from build123d import *

# Parameters (mm, degrees)
BOSS_EXTRUDE1_DEPTH = 20
CUT_EXTRUDE1_DEPTH  = 59.888175724
CUT_EXTRUDE2_DEPTH  = 79.101263393
HOLE1_D             = 3.4
HOLE2_D             = 3.4
HOLE3_D             = 8.4
HOLE4_D             = 8.4
HOLE5_D             = 8.4
CHAMFER1_SIZE       = 8.485281374
CHAMFER2_SIZE       = 5
CHAMFER3_SIZE       = 8.485281374


with BuildPart() as part:
    # Sketch1 → Boss-Extrude1 (new body)
    with BuildSketch(Plane.XY.offset(20)):
        Polygon((15, -34), (15, -11.339745962), (-2.320508076, 18.660254038), (-21.944863729, 29.990381057), (-42.435244785, 24.5), (-36.944863729, 4.009618943), (-15, -8.660254038), (-15, -34), (0, -49), align=None)
    extrude(amount=-BOSS_EXTRUDE1_DEPTH)

    # Sketch2 → Cut-Extrude1 (cut, through all)
    with BuildSketch(Plane(origin=(-7.5, -12.990381057, 0), x_dir=(0.8660254037844394, -0.499999999999999, 0), z_dir=(-0.499999999999999, -0.8660254037844394, 0))):
        with BuildLine():
            Line((-18.978772839, 12.917565156), (-22, 16.046137466))
            Line((-22, 16.046137466), (-25.021227161, 12.917565156))
            ThreePointArc((-25.021227161, 12.917565156), (-22, 5.8), (-18.978772839, 12.917565156))
        make_face()
    extrude(amount=-CUT_EXTRUDE1_DEPTH, mode=Mode.SUBTRACT)

    # Sketch3 → Cut-Extrude2 (cut, through all)
    with BuildSketch(Plane(origin=(15, 0, 0), x_dir=(0, 0, -1), z_dir=(1, 0, 0))):
        with BuildLine():
            Line((-12.917565156, -18.978772839), (-16.046137466, -22))
            Line((-16.046137466, -22), (-12.917565156, -25.021227161))
            ThreePointArc((-12.917565156, -25.021227161), (-5.8, -22), (-12.917565156, -18.978772839))
        make_face()
    extrude(amount=-CUT_EXTRUDE2_DEPTH, mode=Mode.SUBTRACT)

    # Hole1 (through all)
    with Locations(Plane.XY.offset(20)):
        with Locations((0, -12)):
            Hole(HOLE1_D / 2)

    # Hole2 (through all)
    with Locations(Plane.XY.offset(20)):
        with Locations((-10.392304845, 6)):
            Hole(HOLE2_D / 2)

    # Hole3 (through all)
    with Locations(Plane.XY.offset(20)):
        with Locations((-5.412658774, -3.125)):
            Hole(HOLE3_D / 2)

    # Hole4 (through all)
    with Locations(Plane.XY.offset(20)):
        with Locations((-29.444863729, 17)):
            Hole(HOLE4_D / 2)

    # Hole5 (through all)
    with Locations(Plane.XY.offset(20)):
        with Locations((0, -34)):
            Hole(HOLE5_D / 2)

    # Chamfer1
    chamfer1_edges = [part.edges().sort_by_distance(p)[0] for p in [
        (-42.435244785, 24.5, 10),
    ]]
    chamfer(chamfer1_edges, length=CHAMFER1_SIZE)

    # Chamfer2
    chamfer2_edges = [part.edges().sort_by_distance(p)[0] for p in [
        (-15, -8.660254038, 10),
    ]]
    chamfer(chamfer2_edges, length=CHAMFER2_SIZE)

    # Chamfer3
    chamfer3_edges = [part.edges().sort_by_distance(p)[0] for p in [
        (0, -49, 10),
    ]]
    chamfer(chamfer3_edges, length=CHAMFER3_SIZE)


solid = part.part
For this review, take the finished solid that the model builds, in its own axes (mm). A direction names the side the tool comes from. Give positions to 0.01 mm unless a question says otherwise; leave off trailing zeros. Order: outer loops, then holes, each group sorted by start corner. A loop starts at its lowest first (then second) coordinate and runs counter-clockwise, first axis right, second up. Notation, with made-up numbers: M 59,47.5 L 114,47.5 A16 ccw 114,58.5 Z; hole C 18.25,-37.75 d8. An arc over 180 degrees is marked long. Answer in a Markdown table with one row per item. Add a question column.
(1) Consider section A-A on z = 7. State the section outline as (x, y) points (1 decimal).
(2) For faces 5 (the face through (-20.447, 11.563, 14.504)), 6 (the face through (0.21, -23.489, 14.504)), 7 (the face through (15, -22.8, 5.7)), list the 3-axis set-ups (+Z, -Z, +X, -X, +Y, -Y) from which the entire face can be reached by the end or side of a thin tool; tool diameter is ignored.
(3) Consider section B-B on x = 7. State the section outline as (y, z) points, and give its area (3 significant figures).
(4) Consider section C-C on z = 14. State the section outline as (x, y) points (1 decimal), and give its area (3 significant figures).
(5) Consider section D-D on y = 6. Give the number of separate pieces and of enclosed holes in the cut face, and give its area (3 significant figures).
(6) For pin 1 (1.5 mm diameter, centred on y = 5, z = 4, fed in from +X); pin 2 (4 mm diameter, centred on y = 5, z = 17.5, fed in from +X); pin 3 (4 mm diameter, centred on y = 0, z = 15.5, fed in from +X), all flat-tipped, find the tip position at first contact; note any pin that passes through.
(7) Mouldability with a two-part tool opening along X and no side actions: class faces 1 (the face through (0.547, -29.836, 9.86)), 2 (the face through (6.46, 3.45, 10.14)), 3 (the face through (-17.83, 10.05, 14.46)), 4 (the face through (0, -43, 10)) as +X half, -X half, draft (parallel to the pull), parting line (faces both ways), or undercut.
(8) Wall thickness on probe 1 along X at (y, z) = (19, 14.75); probe 2 along Y at (x, z) = (0, 13.25); probe 3 along Y at (x, z) = (-7.25, 10): over which ranges is each line inside the solid? List them lowest first. Write a range as [from, to].
Evaluation:
| question | item | result |
|---|---|---|
| 1 | outline | M -40.2,16.3 L -36.9,4 L -29.1,-0.5 L -14.1,25.5 L -21.9,30 L -34.2,26.7 Z; M -24,-3.5 L -19.3,-6.2 L -15,-13.7 L -15,-19.1 L 15,-19.1 L 15,-11.3 L -2.3,18.7 L -9,22.5 Z; M -15,-34 L -6,-43 L 6,-43 L 15,-34 L 15,-24.9 L -15,-24.9 Z; hole C -29.4,17 d8.4; hole C -10.4,6 d3.4; hole C -5.4,-3.1 d8.4; hole C 0,-34 d8.4; hole C 0,-12 d3.4 |
| 2 | face 5 | none |
| 2 | face 6 | +X, -X |
| 2 | face 7 | +Z, -Z, +X, +Y, -Y |
| 3 | outline | M -42,0 L 2.52,0 L 2.52,20 L -42,20 Z; hole M -25.02,12.92 A4.2 ccw long -18.98,12.92 L -22,16.05 Z |
| 3 | area | 831 mm^2 |
| 4 | outline | M -40.2,16.3 L -36.9,4 L -28.3,-1 L -13.3,25 L -21.9,30 L -34.2,26.7 Z; M -24.8,-3 L -19.3,-6.2 L -15,-13.7 L -15,-20 L 15,-20 L 15,-11.3 L -2.3,18.7 L -9.8,23 Z; M -15,-34 L -6,-43 L 6,-43 L 15,-34 L 15,-24 L -15,-24 Z; hole C -29.4,17 d8.4; hole C -10.4,6 d3.4; hole C -5.4,-3.1 d8.4; hole C 0,-34 d8.4; hole C 0,-12 d3.4 |
| 4 | area | 1,830 mm^2 |
| 5 | separate pieces | 2 |
| 5 | enclosed holes | 1 |
| 5 | area | 713 mm^2 |
| 6 | pin 1 | stops at x = 6 |
| 6 | pin 2 | stops at x = 6.72 |
| 6 | pin 3 | stops at x = 9.61 |
| 7 | face 1 | undercut |
| 7 | face 2 | +X half |
| 7 | face 3 | undercut |
| 7 | face 4 | draft |
| 8 | probe 1 | x = [-38.68, -33.14], [-25.75, -15.88], [-12.99, -2.91] |
| 8 | probe 2 | y = [-43, -38.2], [-29.8, -24.7], [-19.3, -13.7], [-10.3, 14.64] |
| 8 | probe 3 | y = [-41.75, -26.2], [-17.8, -6.9], [0.65, 21.51] |
